from build123d import *

# Parameters (mm, degrees)
ESBO_O1_W                = 25
ESBO_O1_H                = 30
ESBO_O1_W_2              = 40
RESSALTO_EXTRUS_O2_DEPTH = 40
RESSALTO_EXTRUS_O3_DEPTH = 90
ESBO_O3_R                = 16
CORTE_EXTRUS_O1_DEPTH    = 193.093727123
FILETE1_R                = 6
ESBO_O4_W                = 40
ESBO_O4_H                = 30
CORTE_EXTRUS_O2_DEPTH    = 14
CORTE_EXTRUS_O3_DEPTH    = 220.317121995


with BuildPart() as part:
    # Esboço1 → Ressalto-extrusão2 (new body)
    with BuildSketch(Plane(origin=(0, 0, 0), x_dir=(0, 0, -1), z_dir=(1, 0, 0))):
        with Locations((12.5, 15)):
            Rectangle(ESBO_O1_W, ESBO_O1_H)
        with Locations((77.5, 15)):
            Rectangle(ESBO_O1_W, ESBO_O1_H)
        with Locations((45, 15)):
            Rectangle(ESBO_O1_W_2, ESBO_O1_H)
    extrude(amount=RESSALTO_EXTRUS_O2_DEPTH)

    # Esboço2 → Ressalto-extrusão3 (add)
    with BuildSketch(Plane.XY):
        Polygon((40, 30), (40, 120), (110, 120), (110, 104.242681345), (110, 50), (160, 50), (160, 0), (120, 0), (40, 0), align=None)
    extrude(amount=-RESSALTO_EXTRUS_O3_DEPTH)

    # Esboço3 → Corte-extrusão1 (cut, through all)
    with BuildSketch(Plane.ZY.offset(-40)):
        with Locations((-50, 90)):
            Circle(ESBO_O3_R)
    extrude(amount=-CORTE_EXTRUS_O1_DEPTH, mode=Mode.SUBTRACT)

    # Filete1
    filete1_edges = [part.edges().sort_by_distance(p)[0] for p in [
        (75, 120, 0),
    ]]
    fillet(filete1_edges, radius=FILETE1_R)

    # Esboço4 → Corte-extrusão2 (cut)
    with BuildSketch(Plane.ZY):
        with Locations((-45, 15)):
            Rectangle(ESBO_O4_W, ESBO_O4_H)
    extrude(amount=-CORTE_EXTRUS_O2_DEPTH, mode=Mode.SUBTRACT)

    # Esboço5 → Corte-extrusão3 (cut, through all)
    with BuildSketch(Plane.XY):
        Polygon((120, 0), (160, 25), (160, 0), align=None)
    extrude(amount=-CORTE_EXTRUS_O3_DEPTH, mode=Mode.SUBTRACT)


solid = part.part
CAD build for the part. Positions are in the model's coordinates, mm. A direction names the side the tool comes from. Round coordinates to 2 decimals unless told otherwise and drop trailing zeros. Write each loop counter-clockwise with the first axis right and the second up, starting at its lowest first coordinate (ties: lowest second). Pieces come first, ordered by that corner, then holes. Notation, with made-up numbers: M 65.25,80 L 84.25,80 A24 ccw 84.25,93 Z; hole C 89.25,0.5 d11. An arc over 180 degrees is marked long. Use a Markdown table: item, result. Add a question column.
1. Slice it at C-C on x = 79. Give the cut face in (y, z), then the cut area to 3 significant figures.
2. 3-axis set-ups, long thin cutter, end or side, ignore diameter. For faces 1 (the face through (7, 15, -65)), 2 (the face through (135, 50, -44)), 3 (the face through (40, 66, -44)), 4 (the face through (74.51, 105.864, -52.083)), 5 (the face through (0, 15, -77)): which of +Z, -Z, +X, -X, +Y, -Y reach the whole face in a straight line?
3. Flat gauge pins, fed straight in: P1, Ø15, axis at y = 10, z = -53.5, coming from the -X side; P2, Ø1, axis at x = 121.5, z = -78, coming from the +Y side; P3, Ø12, axis at x = 25, z = -60, coming from the +Y side. Where does each tip first touch, or does it go through?
4. Pull direction Z, two halves, no side cores. Call faces 6 (the face through (75, 120, -47)), 7 (the face through (81, 45, 0)), 8 (the face through (14, 15, -45)): released by +Z, released by -Z, zero draft, split by the parting line, or undercut.
5. Slice it at B-B on z = -50. Give the cut face in (x, y).
6. Slice it at A-A on y = 90. Give the cut face in (x, z).
7. Drill centre lines: probe 1 along Y at (x, z) = (92, -50); probe 2 along X at (y, z) = (90, -77.5); probe 3 along Z at (x, y) = (85, 98). Where is each one in solid material? Low to high.
8. Slice it at D-D on z = -22. Give the cut face in (x, y), then the cut area to 3 significant figures.
Reply:
| question | item | result |
|---|---|---|
| 1 | outline | M 0,-90 L 120,-90 L 120,-6 A6 ccw 114,0 L 0,0 Z; hole C 90,-50 d32 |
| 1 | area | 9,990 mm^2 |
| 2 | face 1 | -X, +Y, -Y |
| 2 | face 2 | +Z, -Z, +X, +Y |
| 2 | face 3 | +Z, -Z, -X, +Y |
| 2 | face 4 | +X, -X |
| 2 | face 5 | +Z, -Z, -X, +Y, -Y |
| 3 | P1 | stops at x = 14 |
| 3 | P2 | stops at y = 50 |
| 3 | P3 | stops at y = 30 |
| 4 | face 6 | zero draft |
| 4 | face 7 | released by +Z |
| 4 | face 8 | undercut |
| 5 | outline | M 14,0 L 120,0 L 160,25 L 160,50 L 110,50 L 110,74 L 40,74 L 40,30 L 14,30 Z; M 40,106 L 110,106 L 110,120 L 40,120 Z |
| 6 | outline | M 40,-90 L 110,-90 L 110,-66 L 40,-66 Z; M 40,-34 L 110,-34 L 110,0 L 40,0 Z |
| 7 | probe 1 | y = 0 to 74, 106 to 120 |
| 7 | probe 2 | x = 40 to 110 |
| 7 | probe 3 | z = -90 to -63.86, -36.14 to 0 |
| 8 | outline | M 0,0 L 120,0 L 160,25 L 160,50 L 110,50 L 110,120 L 40,120 L 40,30 L 0,30 Z |
| 8 | area | 11,600 mm^2 |
